Source: CAD feature listing. Evaluate the final solid. Frame: model axes, mm. A direction names the side the tool comes from. Round coordinates to 2 decimals unless told otherwise and drop trailing zeros. Loops run counter-clockwise (first coordinate to the right, second up) from the corner with the lowest first, then second, coordinate; pieces in that order, holes last.
Item 1: Section query A-A on x = -5. Return loops of the section in (y, z).
Item 2: Section query D-D on z = 18.5. Return loops of the section in (x, y), then the cut area to 3 significant figures.
Item 3: Ray query, L1, parallel to X at y = -39.5, z = 6.5; L2, parallel to Z at x = -36, y = -38.15; L3, parallel to X at y = -25.5, z = 21.5. Return the intervals inside material, ascending.
Item 4: Section query C-C on x = -36. Return loops of the section in (y, z).
Item 5: Pull-direction query (X, two-part tool) for faces 1 (the flat face through (-14, -69.5, 12)), 2 (the flat face through (-43.5, -34, 12)), 3 (the flat face through (-1, -85.5, 13)); classes: released by +X, released by -X, zero draft, split by the parting line, or undercut.
Item 6: Section query B-B on y = -79. Return loops of the section in (x, z).
Item 7: First-contact query: P1, Ø10, axis at y = -66.5, z = 17, coming from the -X side; P2, Ø5.5, axis at x = -37, z = 17.5, coming from the -Y side; P3, Ø11, axis at x = -18, z = 12.5, coming from the -Y side. Flat tips, straight axial feed; report the tip coordinate or a pass-through.
Item 8: Access query for faces 4 (the flat face through (-36, -40.25, 12)), 5 (the flat face through (-3, -37, 12)), 6 (the flat face through (-34, -35.25, 12)), 7 (the flat face through (-16, 0, 12)). Directions: +Z, -Z, +X, -X, +Y, -Y. A direction counts if a zero-diameter tool reaches every point of the face in a straight line with its end or side. Return the directions, or none.
```python
from build123d import *

# Parameters (mm, degrees)
BOSS_EXTRUDE1_DEPTH     = 25
SKETCH3_W               = 25
SKETCH3_H               = 13
BOSS_EXTRUDE2_DEPTH     = 3
SKETCH4_R               = 2.15
CUT_EXTRUDE1_DEPTH      = 3
CUT_EXTRUDE2_DEPTH      = 74.16291752
CUT_EXTRUDE2_DEPTH_BACK = 74.16291752
SKETCH5_R               = 2.15


with BuildPart() as part:
    # Sketch2 → Boss-Extrude1 (new body)
    with BuildSketch(Plane.XY):
        Polygon((0, 0), (0, -72.5), (-28.5, -72.5), (-28.5, -40.25), (-43.5, -40.25), (-43.5, -37.25), (-25.5, -37.25), (-25.5, -69.5), (-3, -69.5), (-3, -3), (-25.5, -3), (-25.5, -35.25), (-43.5, -35.25), (-43.5, -32.25), (-28.5, -32.25), (-28.5, 0), align=None)
    extrude(amount=BOSS_EXTRUDE1_DEPTH)

    # Sketch3 → Boss-Extrude2 (add)
    with BuildSketch(Plane(origin=(0, 0, 0), x_dir=(0, 0, -1), z_dir=(1, 0, 0))):
        with Locations((-12.5, 6.5)):
            Rectangle(SKETCH3_W, SKETCH3_H)
        with Locations((-12.5, -79)):
            Rectangle(SKETCH3_W, SKETCH3_H)
    extrude(amount=-BOSS_EXTRUDE2_DEPTH)

    # Sketch4 → Cut-Extrude1 (cut)
    with BuildSketch(Plane.ZY.offset(3)):
        with Locations(Location((12.5, 6.5, 0), (0, 0, 270))):
            Circle(SKETCH4_R)
        with Locations(Location((12.5, -79, 0), (0, 0, 270))):
            Circle(SKETCH4_R)
    extrude(amount=-CUT_EXTRUDE1_DEPTH, mode=Mode.SUBTRACT)

    # Sketch5 → Cut-Extrude2 (cut, two sides: drawn at the far end of the back side and taken through both)
    with BuildSketch(Plane(origin=(0, -32.25, 0), x_dir=(1, 0, 0), z_dir=(0, 1, 0)).offset(-CUT_EXTRUDE2_DEPTH_BACK)):
        with Locations(Location((-36, -6.5, 0), (0, 0, 270))):
            Circle(SKETCH5_R)
        with Locations(Location((-36, -18.5, 0), (0, 0, 270))):
            Circle(SKETCH5_R)
    extrude(amount=CUT_EXTRUDE2_DEPTH + CUT_EXTRUDE2_DEPTH_BACK, mode=Mode.SUBTRACT)


solid = part.part
```
Data:
1. outline: (-72.5, 0) - (-69.5, 0) - (-69.5, 25) - (-72.5, 25) - close; (-3, 0) - (0, 0) - (0, 25) - (-3, 25) - close
2. outline: (-43.5, -40.25) - (-38.15, -40.25) - (-38.15, -37.25) - (-43.5, -37.25) - close; (-43.5, -35.25) - (-38.15, -35.25) - (-38.15, -32.25) - (-43.5, -32.25) - close; (-33.85, -40.25) - (-28.5, -40.25) - (-28.5, -72.5) - (-3, -72.5) - (-3, -85.5) - (0, -85.5) - (0, 13) - (-3, 13) - (-3, 0) - (-28.5, 0) - (-28.5, -32.25) - (-33.85, -32.25) - (-33.85, -35.25) - (-25.5, -35.25) - (-25.5, -3) - (-3, -3) - (-3, -69.5) - (-25.5, -69.5) - (-25.5, -37.25) - (-33.85, -37.25) - close
2. area: 706 mm2
3. L1: x = -43.5 to -38.15, -33.85 to -25.5, -3 to 0
3. L2: z = 0 to 4.35, 8.65 to 16.35, 20.65 to 25
3. L3: x = -28.5 to -25.5, -3 to 0
4. outline: (-40.25, 0) - (-37.25, 0) - (-37.25, 4.35) - (-40.25, 4.35) - close; (-40.25, 8.65) - (-37.25, 8.65) - (-37.25, 16.35) - (-40.25, 16.35) - close; (-40.25, 20.65) - (-37.25, 20.65) - (-37.25, 25) - (-40.25, 25) - close; (-35.25, 0) - (-32.25, 0) - (-32.25, 4.35) - (-35.25, 4.35) - close; (-35.25, 8.65) - (-32.25, 8.65) - (-32.25, 16.35) - (-35.25, 16.35) - close; (-35.25, 20.65) - (-32.25, 20.65) - (-32.25, 25) - (-35.25, 25) - close
5. face 1: undercut
5. face 2: released by -X
5. face 3: zero draft
6. outline: (-3, 0) - (0, 0) - (0, 10.35) - (-3, 10.35) - close; (-3, 14.65) - (0, 14.65) - (0, 25) - (-3, 25) - close
7. P1: stops at x = -28.5
7. P2: stops at y = -40.25
7. P3: stops at y = -72.5
8. face 4: +Z, -Z, -X, -Y
8. face 5: +Z, -Z
8. face 6: +Z, -Z, -X
8. face 7: +Z, -Z, -X, +Y
